Part model, mm, in its own coordinate system. Round coordinates to 2 decimals unless told otherwise and drop trailing zeros. Write each loop counter-clockwise with the first axis right and the second up, starting at its lowest first coordinate (ties: lowest second). Pieces come first, ordered by that corner, then holes. Notation, with made-up numbers: (68, 11) -> (96, 11) arc R14 ccw to (96, 35) -> close; hole circle Ø6 at (-29.5, 78.5). An arc over 180 degrees is marked (long way). Return JSON: item names as keys, results as strings. Group by question number.
```python
from build123d import *

# Parameters (mm, degrees)
SKETCH_W        = 30
SKETCH_H        = 20
PAD_DEPTH       = 20
SKETCH001_W     = 0.5
SKETCH001_H     = 14
POCKET_DEPTH    = 20.001
SKETCH002_R     = 2.1
POCKET001_DEPTH = 30.001
SKETCH003_W     = 0.5
SKETCH003_H     = 14
POCKET002_DEPTH = 26.5


with BuildPart() as part:
    # Sketch → Pad (new body)
    with BuildSketch(Plane.XY):
        Rectangle(SKETCH_W, SKETCH_H)
    extrude(amount=PAD_DEPTH)

    # Sketch001 (on Face2 of Pad) → Pocket (cut, through all)
    with BuildSketch(Plane.XZ.offset(10)):
        with Locations((11.75, 13)):
            Rectangle(SKETCH001_W, SKETCH001_H)
    extrude(amount=-POCKET_DEPTH, mode=Mode.SUBTRACT)

    # Sketch002 (on Face10 of Pocket) → Pocket001 (cut, through all)
    with BuildSketch(Plane.YZ.offset(15)):
        with Locations((0, 10)):
            Circle(SKETCH002_R)
    extrude(amount=-POCKET001_DEPTH, mode=Mode.SUBTRACT)

    # Sketch003 (on Face1 of Pocket001) → Pocket002 (cut)
    with BuildSketch(Plane(origin=(-15, 0, 0), x_dir=(0, -1, 0), z_dir=(-1, 0, 0))):
        with Locations((0, 13)):
            Rectangle(SKETCH003_W, SKETCH003_H)
    extrude(amount=-POCKET002_DEPTH, mode=Mode.SUBTRACT)


solid = part.part
```
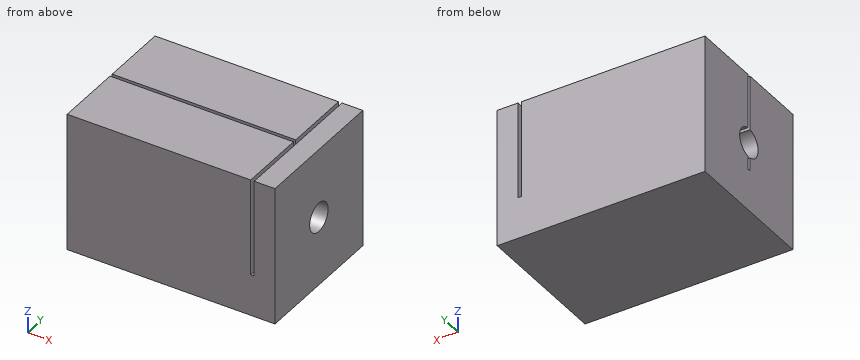
Item 1: Wall check: L1, parallel to Z at x = 13.85, y = 0; L2, parallel to X at y = 5.25, z = 6.25; L3, parallel to Y at x = 2.75, z = 17.5. Give the ranges that are in metal, low to high.
Item 2: Flat gauge pin, fed straight in: P1, Ø5, axis at y = 0, z = 10, coming from the +X side. Where does the tip first touch, or does it go through?
Item 3: Cut at A-A (z = 18.25). Write the cut outline in (x, y), then the cut area to 3 significant figures.
Item 4: Cut at C-C (x = -0.5). Write the cut outline in (y, z).
Item 5: Cut at B-B (z = 10). Write the cut outline in (x, y).
Checks:
{
 "1": {"L1": "z = 0 to 7.9, 12.1 to 20", "L2": "x = -15 to 11.5, 12 to 15", "L3": "y = -10 to -0.25, 0.25 to 10"},
 "2": {"P1": "stops at x = 15"},
 "3": {"outline": "(-15, -10) -> (11.5, -10) -> (11.5, -0.25) -> (-15, -0.25) -> close; (-15, 0.25) -> (11.5, 0.25) -> (11.5, 10) -> (-15, 10) -> close; (12, -10) -> (15, -10) -> (15, 10) -> (12, 10) -> close", "area": "577 mm2"},
 "4": {"outline": "(-10, 0) -> (10, 0) -> (10, 20) -> (0.25, 20) -> (0.25, 12.09) arc R2.1 cw to (0.25, 7.91) -> (0.25, 6) -> (-0.25, 6) -> (-0.25, 7.91) arc R2.1 cw to (-0.25, 12.09) -> (-0.25, 20) -> (-10, 20) -> close"},
 "5": {"outline": "(-15, -10) -> (11.5, -10) -> (11.5, -2.1) -> (-15, -2.1) -> close; (-15, 2.1) -> (11.5, 2.1) -> (11.5, 10) -> (-15, 10) -> close; (12, -10) -> (15, -10) -> (15, -2.1) -> (12, -2.1) -> close; (12, 2.1) -> (15, 2.1) -> (15, 10) -> (12, 10) -> close"}
}
